Design review of the part shown in the three views and the two pictorial views. Dimensions are in mm from the part's minimum x, y and z. A direction names the side the tool comes from. Round coordinates to 2 decimals unless told otherwise and drop trailing zeros. Loops run counter-clockwise (first coordinate to the right, second up) from the corner with the lowest first, then second, coordinate; pieces in that order, holes last. Notation, with made-up numbers: (80.25, 55.25) - (90.25, 55.25) arc R9 cw to (90.25, 65.25) - close; hole circle Ø7 at (-29, -17.75). An arc over 180 degrees is marked (long way). Return JSON: item names as keys, results as strings. Group by question number.
(1) Wall thickness on L1, parallel to Y at x = 63.5, z = 5.25; L2, parallel to X at y = 14.5, z = 5; L3, parallel to X at y = 15.5, z = 4: over which ranges is each line inside the solid? List them lowest first. Write a range as [from, to].
(2) We need section A-A, the plane y = 8.25. Write out the cut boundary in (x, z).
(3) For the marked faces 4 and 5, list the 3-axis set-ups (+Z, -Z, +X, -X, +Y, -Y) from which the entire face can be reached by the end or side of a thin tool; tool diameter is ignored.
(4) The part is to be moulded in two halves that separate along X. For the marked faces 1, 2 and 3, say which applies: pulls with the +X half, pulls with the -X half, needs draft (parallel to the pull), parting line crosses it, or undercut.
(5) We need section B-B, the plane z = 34. Write out the cut boundary in (x, y), and give its area (3 significant figures).
(6) We need section C-C, the plane x = 10. Write out the cut boundary in (y, z), and give its area (3 significant figures).
(7) We need section D-D, the plane x = 29.5. Write out the cut boundary in (y, z).
(8) Clearance check with flat-ended pins moving along their axes: pin 1 (6 mm diameter, centred on y = 16, z = 35, fed in from +X); pin 2 (6 mm diameter, centred on y = 11, z = 18, fed in from -X); pin 3 (7.5 mm diameter, centred on x = 8.5, y = 15.5, fed in from +Z). State where each tip first meets the part, or that it passes through.
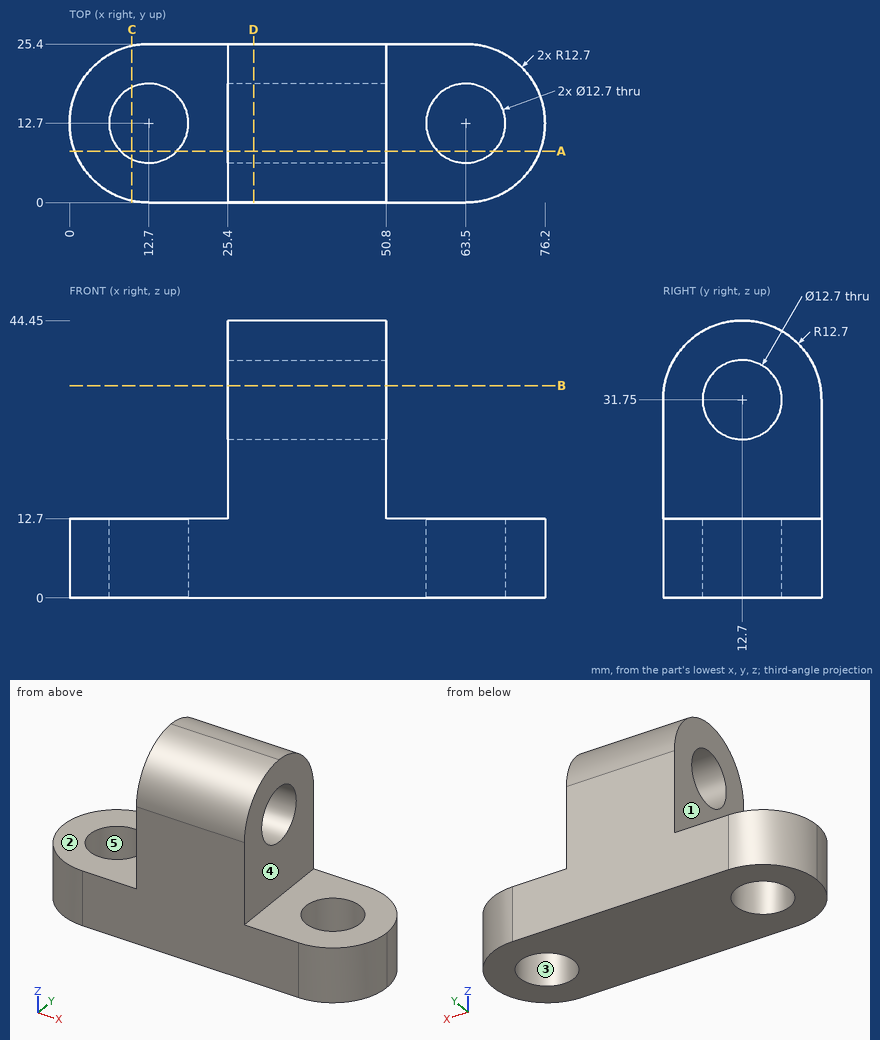
Solutions:
{
 "1": {"L1": "[0, 6.35], [19.05, 25.4]", "L2": "[0.13, 6.61], [18.79, 57.41], [69.59, 76.07]", "L3": "[0.31, 7], [18.4, 57.8], [69.2, 75.89]"},
 "2": {"outline": "(0.81, 0) - (8.17, 0) - (8.17, 12.7) - (0.81, 12.7) - close; (17.23, 0) - (58.97, 0) - (58.97, 12.7) - (50.8, 12.7) - (50.8, 27.22) - (25.4, 27.22) - (25.4, 12.7) - (17.23, 12.7) - close; (25.4, 36.28) - (50.8, 36.28) - (50.8, 43.64) - (25.4, 43.64) - close; (68.03, 0) - (75.39, 0) - (75.39, 12.7) - (68.03, 12.7) - close"},
 "3": {"face 4": "+Z, +X, +Y, -Y", "face 5": "+Z, -Z"},
 "4": {"face 1": "pulls with the -X half", "face 2": "needs draft", "face 3": "undercut"},
 "5": {"outline": "(25.4, 0.2) - (50.8, 0.2) - (50.8, 6.76) - (25.4, 6.76) - close; (25.4, 18.64) - (50.8, 18.64) - (50.8, 25.2) - (25.4, 25.2) - close", "area": "333 mm^2"},
 "6": {"outline": "(0.29, 0) - (6.95, 0) - (6.95, 12.7) - (0.29, 12.7) - close; (18.45, 0) - (25.11, 0) - (25.11, 12.7) - (18.45, 12.7) - close", "area": "169 mm^2"},
 "7": {"outline": "(0, 0) - (25.4, 0) - (25.4, 31.75) arc R12.7 ccw to (0, 31.75) - close; hole circle Ø12.7 at (12.7, 31.75)"},
 "8": {"pin 1": "x = 50.8", "pin 2": "x = 25.4", "pin 3": "z = 12.7"}
}
